from build123d import *

# Parameters (mm, degrees)
F0_W          = 10
F0_H          = 40
F1_DEPTH      = 7
F1_DEPTH_BACK = 7
F2_R          = 1
F3_DEPTH      = 4


with BuildPart() as f1:
    # F0 (on Right) → F1 (new body, two sides)
    with BuildSketch(Plane.YZ) as f1_sk:
        Rectangle(F0_W, F0_H)
    extrude(amount=F1_DEPTH)
    extrude(f1_sk.sketch, amount=-F1_DEPTH_BACK)

    # F2 (on face) → F3 (join)
    with BuildSketch(Plane.XZ.offset(5)):
        with Locations((0, 8)):
            Circle(F2_R)
        with Locations((0, -8)):
            Circle(F2_R)
    extrude(amount=F3_DEPTH)


solid = f1.part
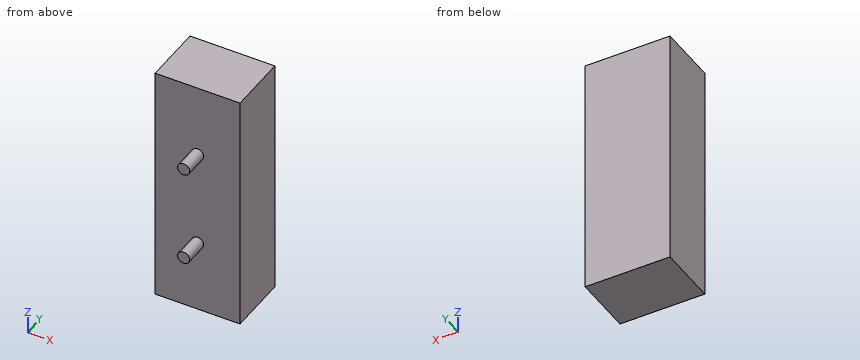
CAD build for the part. Positions are in the model's coordinates, mm. Round coordinates to 2 decimals unless told otherwise and drop trailing zeros. Write each loop counter-clockwise with the first axis right and the second up, starting at its lowest first coordinate (ties: lowest second). Pieces come first, ordered by that corner, then holes.
(1) Slice it at A-A, the plane x = 0. Write the cut outline in (y, z), and give its area (3 significant figures).
(2) Slice it at C-C, the plane z = 8. Write the cut outline in (x, y), and give its area (3 significant figures).
(3) Slice it at D-D, the plane z = -6.5. Write the cut outline in (x, y).
(4) Probe line 1 along Y through (x, z) = (-5.25, -7). List the from-to ranges inside material, lowest first.
(5) Slice it at B-B, the plane y = -5.5. Write the cut outline in (x, z).
From the geometry:
1. outline: (-9, -9) - (-5, -9) - (-5, -20) - (5, -20) - (5, 20) - (-5, 20) - (-5, 9) - (-9, 9) - (-9, 7) - (-5, 7) - (-5, -7) - (-9, -7) - close
1. area: 416 mm2
2. outline: (-7, -5) - (-1, -5) - (-1, -9) - (1, -9) - (1, -5) - (7, -5) - (7, 5) - (-7, 5) - close
2. area: 148 mm2
3. outline: (-7, -5) - (7, -5) - (7, 5) - (-7, 5) - close
4. line 1: y = -5 to 5
5. outline: circle Ø2 at (0, -8); circle Ø2 at (0, 8)
